Build history of the part. All positions in model axes, mm. Coordinates: 2 decimals unless noted, no trailing zeros. Order: outer loops, then holes, each group sorted by start corner. A loop starts at its lowest first (then second) coordinate and runs counter-clockwise, first axis right, second up. Notation, with made-up numbers: (-12.5, -22.5) - (42.5, -22.5) arc R15 cw to (42.5, -8.5) - close; hole circle Ø10 at (48, -24). An arc over 180 degrees is marked (long way). Write each question's results on one line, items separated by ' | '.
Solid Edge part; units mm, degrees
sketch "Sketch1" plane through (0, 0, 0) normal (0, 0, 1) x (1, 0, 0)
  circle A0 centre (31.04, -15.72) radius 1.6
  circle A1 centre (-19.76, -20.8) radius 1.6
  line L0 (-35, -30) -> (-35, 30)
  line L1 (-35, 30) -> (35, 30)
  line L2 (35, 30) -> (35, -30)
  line L3 (35, -30) -> (-35, -30)
  circle A2 centre (31.04, 12.22) radius 1.6
  circle A3 centre (-19.76, 27.46) radius 1.6
extrude "Protrusion1" add sketch "Sketch1" along normal blind 2
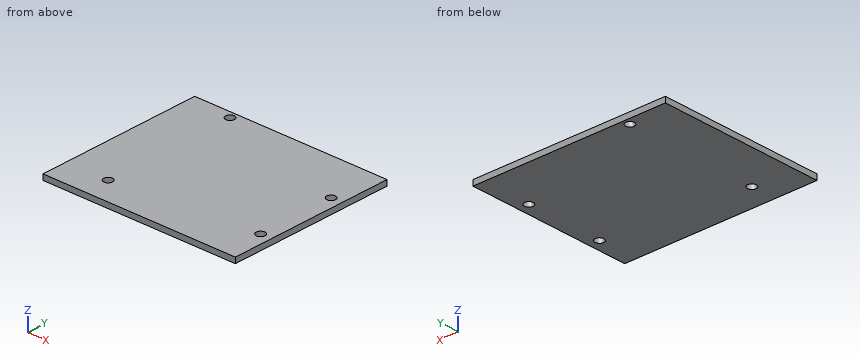
1. Band-saw the part on B-B on y = -15.72. Give the cut face in (x, z).
Solved:
outline: (-35, 0) - (29.44, 0) - (29.44, 2) - (-35, 2) - close; (32.64, 0) - (35, 0) - (35, 2) - (32.64, 2) - close
2. Drop a flat-ended pin along its axis: pin 1 Ø1.5 at (x, y) = (15.5, -13) entering from -Z. Give the stop position or say it passes through.
Solved:
pin 1: stops at z = 0
3. Probe line 1 (Y direction, x = -20, z = 0.65); line 2 (Y direction, x = -19.76, z = 0.9); line 3 (X direction, y = -15.5, z = 0.25). List the from-to ranges inside material, lowest first.
Solved:
line 1: y = -30 to -22.38, -19.22 to 25.88, 29.04 to 30 | line 2: y = -30 to -22.4, -19.2 to 25.86, 29.06 to 30 | line 3: x = -35 to 29.46, 32.62 to 35
4. Band-saw the part on A-A on x = -19.76. Give the cut face in (y, z), then the cut area to 3 significant figures.
Solved:
outline: (-30, 0) - (-22.4, 0) - (-22.4, 2) - (-30, 2) - close; (-19.2, 0) - (25.86, 0) - (25.86, 2) - (-19.2, 2) - close; (29.06, 0) - (30, 0) - (30, 2) - (29.06, 2) - close | area: 107 mm2
